from build123d import *

# Parameters (mm, degrees)
F0_W     = 40
F0_H     = 5
F1_DEPTH = 20
F3_D     = 5
F5_D     = 5
F6_R     = 10


# Not quite as in the source:
# - a feature names something its author has since deleted; it is built from what else it names


with BuildPart() as f1:
    # F0 (on Front) → F1 (new body)
    with BuildSketch(Plane.XZ):
        Polygon((19.9351918133, 52), (19.9351918133, 10), (24.9351918133, 10), (24.9351918133, 90), (19.9351918133, 90), (19.9351918133, 55), align=None)
        with Locations((-5.0648081867, 2.5)):
            Rectangle(F0_W, F0_H)
        with BuildLine():
            ThreePointArc((19.9351918133, 10), (18.4707257193, 6.4644660941), (14.9351918133, 5))
            Line((14.9351918133, 5), (14.9351918133, 0))
            ThreePointArc((14.9351918133, 0), (22.0062596252, 2.9289321881), (24.9351918133, 10))
            Line((24.9351918133, 10), (19.9351918133, 10))
        make_face()
        Polygon((16.9351918133, 55), (19.9351918133, 55), (19.9351918133, 90), (19.9351918133, 95), (16.9351918133, 95), align=None)
        with BuildLine():
            Line((19.9351918133, 90), (24.9351918133, 90))
            ThreePointArc((24.9351918133, 90), (23.4707257193, 93.5355339059), (19.9351918133, 95))
            Line((19.9351918133, 95), (19.9351918133, 90))
        make_face()
        with BuildLine():
            ThreePointArc((16.9351918133, 55), (19.0565121569, 54.1213203436), (19.9351918133, 52))
            Line((19.9351918133, 52), (19.9351918133, 55))
            Line((19.9351918133, 55), (16.9351918133, 55))
        make_face()
    extrude(amount=F1_DEPTH)

    # F3 (through all)
    with Locations(Plane(origin=(0, 0, 0), x_dir=(0, 1, 0), z_dir=(-1, 0, 0))):
        with Locations((-10, -85), (-10, -65)):
            Hole(F3_D / 2)

    # F5 (through all)
    with Locations(Plane(origin=(0, 0, 0), x_dir=(1, 0, 0), z_dir=(0, 0, -1))):
        with Locations((-15.0648081867, 10), (4.9351918133, 10)):
            Hole(F5_D / 2)

    # F6
    f6_edges = [f1.edges().sort_by_distance(p)[0] for p in [
        (-25.064808, -20, 2.5),
    ]]
    fillet(f6_edges, radius=F6_R)


solid = f1.part
Input: part model. Units: mm. Frame: model coordinates. A direction names the side the tool comes from. Coordinates: 2 decimals unless noted, no trailing zeros. Loops run counter-clockwise (first coordinate to the right, second up) from the corner with the lowest first, then second, coordinate; pieces in that order, holes last. Notation, with made-up numbers: (0.5, 70) -> (56.5, 70) arc R24 cw to (56.5, 82) -> close; hole circle Ø9 at (70.25, -11). An arc over 180 degrees is marked (long way). Write each question's results on one line, items separated by ' | '. Start each with the question number.
Q1. Pull-direction query (X, two-part tool) for faces 1 (the cylindrical face through (-14.52, -7.56, 2.53)), 2 (the cylindrical face through (20.99, -9.67, 82.52)), 3 (the cylindrical face through (23.509, -9.86, 93.496)); classes: released by +X, released by -X, zero draft, split by the parting line, or undercut.
Q2. Section D-D, the plane y = -11.5. Return the cut outline in (x, z), plus the area to 3 significant figures.
Q3. Reachability of faces 4 (the flat face through (-25.065, -5, 2)), 5 (the flat face through (-5, -10, 5)), 6 (the cylindrical face through (18.509, -9.86, 6.504)) from +Z, -Z, +X, -X, +Y, -Y: full face, straight path, thin tool, end or side. Return the list, or none.
Q4. Ray query, line 1 (Y direction, x = 21.25, z = 85); line 2 (X direction, y = -10, z = 3.4); line 3 (Z direction, x = 18.75, y = -10). Return the intervals inside material, ascending. Write a range as from..to.
Q5. Section B-B, the plane y = -6. Return the cut outline in (x, z), plus the area to 3 significant figures.
Q6. Section A-A, the plane z = 65. Return the cut outline in (x, y), plus the area to 3 significant figures.
Q7. Pin query (flat end, axial travel): pin 1 (6 mm diameter, centred on y = -12.5, z = 21, fed in from -X). Return the tip coordinate at first contact, or that it passes through.
Q8. Section C-C, the plane x = -16. Return the cut outline in (y, z).
Found:
1) face 1: undercut | face 2: zero draft | face 3: released by +X
2) outline: (-24.95, 0) -> (-17.06, 0) -> (-17.06, 5) -> (-24.95, 5) -> close; (-13.06, 0) -> (2.94, 0) -> (2.94, 5) -> (-13.06, 5) -> close; (6.94, 0) -> (14.94, 0) arc R10 ccw to (24.94, 10) -> (24.94, 63) -> (16.94, 63) -> (16.94, 55) arc R3 cw to (19.94, 52) -> (19.94, 10) arc R5 cw to (14.94, 5) -> (6.94, 5) -> close; (16.94, 67) -> (24.94, 67) -> (24.94, 83) -> (16.94, 83) -> close; (16.94, 87) -> (24.94, 87) -> (24.94, 90) arc R5 ccw to (19.94, 95) -> (16.94, 95) -> close | area: 696 mm2
3) face 4: +Z, -Z, -X, +Y, -Y | face 5: +Z, -X, +Y, -Y | face 6: -X, +Y, -Y
4) line 1: -20..-12.5, -7.5..0 | line 2: -25.06..-17.56, -12.56..2.44, 7.44..22.45 | line 3: 0.76..6.77, 54.39..62.5, 67.5..82.5, 87.5..95
5) outline: (-25.06, 0) -> (14.94, 0) arc R10 ccw to (24.94, 10) -> (24.94, 90) arc R5 ccw to (19.94, 95) -> (16.94, 95) -> (16.94, 55) arc R3 cw to (19.94, 52) -> (19.94, 10) arc R5 cw to (14.94, 5) -> (-25.06, 5) -> close | area: 800 mm2
6) outline: (16.94, -20) -> (24.94, -20) -> (24.94, -12.5) -> (16.94, -12.5) -> close; (16.94, -7.5) -> (24.94, -7.5) -> (24.94, 0) -> (16.94, 0) -> close | area: 120 mm2
7) pin 1: x = 19.94
8) outline: (-19.96, 0) -> (-12.32, 0) -> (-12.32, 5) -> (-19.96, 5) -> close; (-7.68, 0) -> (0, 0) -> (0, 5) -> (-7.68, 5) -> close
